Design review of the part built by this model. Coordinates are the model's own, in mm. A direction names the side the tool comes from. Give positions to 0.01 mm unless a question says otherwise; leave off trailing zeros. Loops run counter-clockwise (first coordinate to the right, second up) from the corner with the lowest first, then second, coordinate; pieces in that order, holes last. Notation, with made-up numbers: (29.5, 36) -> (80.5, 36) arc R17 cw to (80.5, 69) -> close; hole circle Ø4 at (77, 62). An arc over 180 degrees is marked (long way). Use a Markdown table: item, result. Add a question column.
1. Add section C-C (z = 12). State the section outline as (x, y) points, and give its area (3 significant figures).
2. Draft analysis for pull direction X (two halves, no side actions). For faces 1 (the cylindrical face through (11.923, 3.755, 30.927)), 2 (the cylindrical face through (-87.5, 0.1, -4.9)), 3 (the flat face through (0, 125, 81)), 4 (the cylindrical face through (-54, 0, -5)), state which applies: pulls with the +X half, pulls with the -X half, needs draft (parallel to the pull), parting line crosses it, or undercut.
3. Add section D-D (y = 80). State the section outline as (x, z) points.
4. Add section B-B (x = -21.5). State the section outline as (y, z) points, and give its area (3 significant figures).
5. To check wall thickness, follow line 1 (X direction, y = 0, z = -5.5); line 2 (Y direction, x = -60, z = -3.75); line 3 (Z direction, x = -83, y = 7). State the ranges of each line that lie inside material, in increasing order.
6. For faces 5 (the cylindrical face through (-115.233, 1.341, -14.93)), 6 (the flat face through (-74, -4.5, -5)), 7 (the cylindrical face through (6.72, 73.24, 70.46)), list the 3-axis set-ups (+Z, -Z, +X, -X, +Y, -Y) from which the entire face can be reached by the end or side of a thin tool; tool diameter is ignored.
7. For pin 1 Ø1 at (x, y) = (-16.5, 0.5) entering from -Z; pin 2 Ø1.5 at (y, z) = (6, 33.5) entering from -X; pin 3 Ø5 at (x, z) = (-78, -6.5) entering from +Y, all flat-tipped, find the tip position at first contact; note any pin that passes through.
8. Add section A-A (x = -60). State the section outline as (y, z) points, and give its area (3 significant figures).
Autodesk Inventor part; units mm, degrees
ref_plane "Work Plane1" through (0, 0, 61) normal (0, 0, 1) x (1, 0, 0)
ref_plane "YZ Plane" through (0, 0, 0) normal (1, 0, 0) x (0, 1, 0)
ref_plane "XZ Plane" through (0, 0, 0) normal (0, 1, 0) x (-1, 0, 0)
sketch "Sketch1" plane through (0, 0, 0) normal (0, 0, 1) x (1, 0, 0)
  circle A0 centre (0, 0) radius 12.5
  dimension "d0" = 25
sketch "Sketch2" plane through (0, 0, 0) normal (1, 0, 0) x (0, 1, 0)
  line L0 (0, 0) -> (0, 61)
  arc A0 (20, 81) -> (0, 61) centre (20, 61) ccw
  line L1 (20, 81) -> (125, 81)
  dimension "d1" = 61
  dimension "d30" = 105
  dimension "d31" = 20
ref_plane "Work Plane1" through (0, 0, 61) normal (0, 0, 1) x (1, 0, 0)
sweep "Sweep2" add profiles "Sketch1" path "Sketch2"
sketch "Sketch4" plane through (0, 0, 0) normal (0, 0, -1) x (-1, 0, 0)
  line L0 (-66, 0) -> (120, 0) construction
  line L1 (-66, 22) -> (120, 22)
  line L2 (120, -22) -> (-66, -22)
  arc A0 (-66, 22) -> (-66, -22) centre (-66, 0) ccw
  arc A1 (120, -22) -> (120, 22) centre (120, 0) ccw
  circle A2 centre (0, 0) radius 12.5
  point P0 (27, 0)
  point P1 (27, 0)
  point P2 (142, 0)
  point P3 (-88, 0)
  dimension "d10" = 44
  dimension "d12" = 88
  dimension "d13" = 230
extrude "Extrusion1" add sketch "Sketch4" along normal blind 10 contours L1 A1 L2 A0 | A2
sketch "Sketch5" plane through (0, 0, -10) normal (0, 0, -1) x (-1, 0, 0)
  circle A0 centre (-75, 0) radius 3.5
  circle A1 centre (21.5, 0) radius 3.5
  circle A2 centre (112, 0) radius 3.5
  circle A3 centre (0, 0) radius 12.5
  dimension "d16" = 7
  dimension "d17" = 21.5
  dimension "d18" = 75
  dimension "d19" = 90.5
extrude "Extrusion2" add sketch "Sketch5" along normal blind 10 contours A0 | A1 | A2
sketch "Sketch6" plane through (0, 0, 0) normal (0, 0, 1) x (1, 0, 0)
  arc A0 (-63.9686, -4.5) -> (-63.9686, 4.5) centre (-60, 0) ccw
  circle A1 centre (0, 0) radius 12.5
  line L0 (-63.9686, 4.5) -> (-83, 4.5)
  arc A2 (-83, 4.5) -> (-83, -4.5) centre (-83, 0) ccw
  line L1 (-83, -4.5) -> (-63.9686, -4.5)
  arc A3 (-120, 22) -> (-120, -22) centre (-120, 0) ccw
  point P0 (-142, 0)
  dimension "d22" = 12
  dimension "d23" = 60
  dimension "d24" = 4.5
  dimension "d25" = 23
extrude "Extrusion3" cut sketch "Sketch6" against normal blind 10 contours L1 A2 L0 A0
properties part number "garnitur_lang"
Taken from the geometry:
| question | item | result |
|---|---|---|
| 1 | outline | circle Ø25 at (0, 0) |
| 1 | area | 491 mm^2 |
| 2 | face 1 | parting line crosses it |
| 2 | face 2 | undercut |
| 2 | face 3 | needs draft |
| 2 | face 4 | undercut |
| 3 | outline | circle Ø25 at (0, 81) |
| 4 | outline | (-22, -10) -> (-3.5, -10) -> (-3.5, -20) -> (3.5, -20) -> (3.5, -10) -> (22, -10) -> (22, 0) -> (-22, 0) -> close |
| 4 | area | 510 mm^2 |
| 5 | line 1 | x = -142 to -87.5, -54 to 88 |
| 5 | line 2 | y = -22 to -6, 6 to 22 |
| 5 | line 3 | z = -10 to 0 |
| 6 | face 5 | -Z |
| 6 | face 6 | +Z, -Z |
| 6 | face 7 | +Y |
| 7 | pin 1 | stops at z = -10 |
| 7 | pin 2 | stops at x = -11.34 |
| 7 | pin 3 | stops at y = 22 |
| 8 | outline | (-22, -10) -> (-6, -10) -> (-6, 0) -> (-22, 0) -> close; (6, -10) -> (22, -10) -> (22, 0) -> (6, 0) -> close |
| 8 | area | 320 mm^2 |
